```python
from build123d import *

# Parameters (mm, degrees)
SKETCH_1_R               = 36
EXTRUDE_1_DEPTH          = 43
SKETCH_2_R               = 34
CUT_EXTRUDE_1_DEPTH      = 1.5
SKETCH_5_R               = 32.5
CUT_EXTRUDE_2_DEPTH      = 38.3
SKETCH_6_R               = 21.2
EXTRUDE_2_DEPTH          = 2.6
SKETCH_6_3_R             = 20
CUT_EXTRUDE_3_DEPTH      = 7
CUT_EXTRUDE_3_DEPTH_BACK = 8.6
CUT_EXTRUDE_4_DEPTH      = 37
CUT_EXTRUDE_5_DEPTH      = 3


with BuildPart() as part:
    # Sketch 1 → Extrude 1 (new body)
    with BuildSketch(Plane.XY):
        Circle(SKETCH_1_R)
    extrude(amount=EXTRUDE_1_DEPTH)

    # Sketch 2 → Cut-Extrude 1 (cut)
    with BuildSketch(Plane.XY.offset(43)):
        Circle(SKETCH_2_R)
    extrude(amount=-CUT_EXTRUDE_1_DEPTH, mode=Mode.SUBTRACT)

    # Sketch 5 → Cut-Extrude 2 (cut)
    with BuildSketch(Plane(origin=(0, 0, 0), x_dir=(-1, 0, 0), z_dir=(0, 0, -1))):
        Circle(SKETCH_5_R)
    extrude(amount=-CUT_EXTRUDE_2_DEPTH, mode=Mode.SUBTRACT)

    # Sketch 6 → Extrude 2 (add)
    with BuildSketch(Plane(origin=(0, 0, 38.3), x_dir=(-1, 0, 0), z_dir=(0, 0, -1))):
        Circle(SKETCH_6_R)
    extrude(amount=EXTRUDE_2_DEPTH)

    # Sketch 6_3 → Cut-Extrude 3 (cut, two sides)
    with BuildSketch(Plane(origin=(0, 0, 38.3), x_dir=(-1, 0, 0), z_dir=(0, 0, -1))) as cut_extrude_3_sk:
        Circle(SKETCH_6_3_R)
    extrude(amount=CUT_EXTRUDE_3_DEPTH, mode=Mode.SUBTRACT)
    extrude(cut_extrude_3_sk.sketch, amount=-CUT_EXTRUDE_3_DEPTH_BACK, mode=Mode.SUBTRACT)

    # Sketch 3 → Cut-Extrude 4 (cut, through all)
    with BuildSketch(Plane(origin=(0, 0, 0), x_dir=(1, 0, 0), z_dir=(0, 1, 0))):
        with BuildLine():
            ThreePointArc((11.100980486, 0), (9.326403912, -2.499387259), (8.7, -5.5))
            ThreePointArc((8.7, -5.5), (16.2, -13), (23.7, -5.5))
            ThreePointArc((23.7, -5.5), (23.073596088, -2.499387259), (21.299019514, 0))
            Line((21.299019514, 0), (11.100980486, 0))
        make_face()
        with BuildLine():
            ThreePointArc((21.299019514, 0), (16.2, 2), (11.100980486, 0))
            Line((11.100980486, 0), (21.299019514, 0))
        make_face()
        with BuildLine():
            ThreePointArc((21.299019514, 0), (23.073596088, -2.499387259), (23.7, -5.5))
            Line((23.7, -5.5), (23.7, 0))
            Line((23.7, 0), (21.299019514, 0))
        make_face()
        with BuildLine():
            Line((8.7, 0), (8.7, -5.5))
            ThreePointArc((8.7, -5.5), (9.326403912, -2.499387259), (11.100980486, 0))
            Line((11.100980486, 0), (8.7, 0))
        make_face()
        with BuildLine():
            Line((-23.7, 0), (-23.7, -5.5))
            ThreePointArc((-23.7, -5.5), (-23.073596088, -2.499387259), (-21.299019514, 0))
            Line((-21.299019514, 0), (-23.7, 0))
        make_face()
        with BuildLine():
            ThreePointArc((-21.299019514, 0), (-23.073596088, -2.499387259), (-23.7, -5.5))
            ThreePointArc((-23.7, -5.5), (-16.2, -13), (-8.7, -5.5))
            ThreePointArc((-8.7, -5.5), (-9.326403912, -2.499387259), (-11.100980486, 0))
            Line((-11.100980486, 0), (-21.299019514, 0))
        make_face()
        with BuildLine():
            ThreePointArc((-11.100980486, 0), (-16.2, 2), (-21.299019514, 0))
            Line((-21.299019514, 0), (-11.100980486, 0))
        make_face()
        with BuildLine():
            ThreePointArc((-11.100980486, 0), (-9.326403912, -2.499387259), (-8.7, -5.5))
            Line((-8.7, -5.5), (-8.7, 0))
            Line((-8.7, 0), (-11.100980486, 0))
        make_face()
    extrude(amount=-CUT_EXTRUDE_4_DEPTH, mode=Mode.SUBTRACT)

    # Sketch 7 → Cut-Extrude 5 (cut)
    with BuildSketch(Plane(origin=(0, 0, 38.3), x_dir=(-1, 0, 0), z_dir=(0, 0, -1))):
        with BuildLine():
            Line((-8.7, -18.008609052), (-8.7, -19.332614929))
            ThreePointArc((-8.7, -19.332614929), (0, -21.2), (8.7, -19.332614929))
            Line((8.7, -19.332614929), (8.7, -18.008609052))
            ThreePointArc((8.7, -18.008609052), (0, -20), (-8.7, -18.008609052))
        make_face()
    extrude(amount=CUT_EXTRUDE_5_DEPTH, mode=Mode.SUBTRACT)


solid = part.part
```
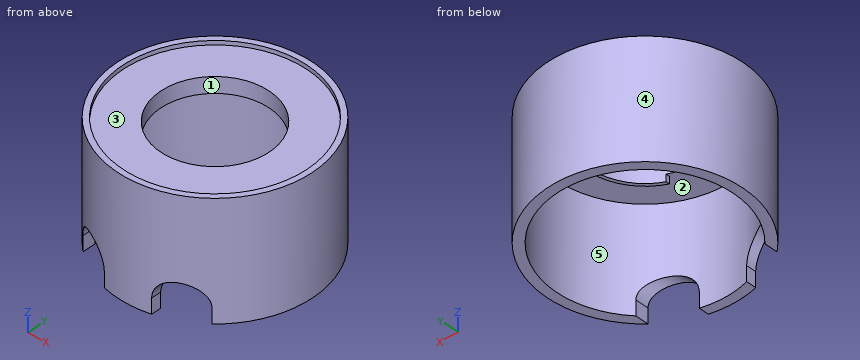
For this review, take the finished solid that the model builds, in its own axes (mm). Face numbers are marked on the shaded views. A direction names the side the tool comes from. Coordinates: 2 decimals unless noted, no trailing zeros. Loops run counter-clockwise (first coordinate to the right, second up) from the corner with the lowest first, then second, coordinate; pieces in that order, holes last. Notation, with made-up numbers: (40, 87) -> (93, 87) arc R15 cw to (93, 106) -> close; hole circle Ø6 at (9.25, 43). An arc over 180 degrees is marked (long way). Return JSON: item names as keys, results as strings. Group by question number.
(1) Mouldability with a two-part tool opening along Y and no side actions: class the marked faces 4 and 5 as pulls with the +Y half, pulls with the -Y half, needs draft (parallel to the pull), parting line crosses it, or undercut.
(2) Consider section B-B, the plane x = 0. Give the boundary of the cut face in (y, z), plus the area to 3 significant figures.
(3) Consider section C-C, the plane z = 23.5. Give the boundary of the cut face in (x, y), plus the area to 3 significant figures.
(4) Consider section D-D, the plane x = -12.5. Give the boundary of the cut face in (y, z).
(5) For pin 1 Ø1.5 at (x, z) = (26, 28) entering from -Y; pin 2 Ø4 at (y, z) = (-24, 4) entering from -X; pin 3 Ø12 at (x, y) = (-24.5, 2) entering from -Z; pin 4 Ø24 at (x, y) = (0, 0) entering from -Z, all flat-tipped, find the tip position at first contact; note any pin that passes through.
(6) Consider section A-A, the plane y = 0. Give the boundary of the cut face in (x, z).
(7) Tool access review of the marked faces 1, 2 and 3: name each direction out of +Z, -Z, +X, -X, +Y, -Y from which nothing blocks a thin tool from reaching the whole face with its end or side.
(8) To check wall thickness, follow L1, parallel to X at y = 0, z = 36.9; L2, parallel to Y at x = -13, z = 36.5; L3, parallel to X at y = 0, z = 39. State the ranges of each line that lie inside material, in increasing order.
Results below:
{
 "1": {"face 4": "parting line crosses it", "face 5": "undercut"},
 "2": {"outline": "(-36, 0) -> (-32.5, 0) -> (-32.5, 38.3) -> (-20, 38.3) -> (-20, 41.5) -> (-34, 41.5) -> (-34, 43) -> (-36, 43) -> close; (20, 35.7) -> (21.2, 35.7) -> (21.2, 38.3) -> (32.5, 38.3) -> (32.5, 0) -> (36, 0) -> (36, 43) -> (34, 43) -> (34, 41.5) -> (20, 41.5) -> close", "area": "380 mm2"},
 "3": {"outline": "circle Ø72 at (0, 0); hole circle Ø65 at (0, 0)", "area": "753 mm2"},
 "4": {"outline": "(-33.76, 12.02) -> (-30, 12.02) -> (-30, 38.3) -> (-17.12, 38.3) -> (-17.12, 35.7) -> (-15.61, 35.7) -> (-15.61, 41.5) -> (-31.62, 41.5) -> (-31.62, 43) -> (-33.76, 43) -> close; (15.61, 35.7) -> (17.12, 35.7) -> (17.12, 38.3) -> (30, 38.3) -> (30, 0) -> (33.76, 0) -> (33.76, 43) -> (31.62, 43) -> (31.62, 41.5) -> (15.61, 41.5) -> close"},
 "5": {"pin 1": "stops at y = -25.66", "pin 2": "stops at x = -28.5", "pin 3": "stops at z = 35.7", "pin 4": "passes through"},
 "6": {"outline": "(-36, 0) -> (-32.5, 0) -> (-32.5, 38.3) -> (-21.2, 38.3) -> (-21.2, 35.7) -> (-20, 35.7) -> (-20, 41.5) -> (-34, 41.5) -> (-34, 43) -> (-36, 43) -> close; (20, 35.7) -> (21.2, 35.7) -> (21.2, 38.3) -> (32.5, 38.3) -> (32.5, 0) -> (36, 0) -> (36, 43) -> (34, 43) -> (34, 41.5) -> (20, 41.5) -> close"},
 "7": {"face 1": "+Z, -Z", "face 2": "-Z", "face 3": "+Z"},
 "8": {"L1": "x = -36 to -32.5, -21.2 to -20, 20 to 21.2, 32.5 to 36", "L2": "y = -33.57 to -29.79, -16.75 to -15.2, 15.2 to 16.75, 29.79 to 33.57", "L3": "x = -36 to -20, 20 to 36"}
}
